The listing builds one solid part. Answer for the finished solid, in the listing's coordinates (mm). A direction names the side the tool comes from. Round coordinates to 2 decimals unless told otherwise and drop trailing zeros. Write each loop counter-clockwise with the first axis right and the second up, starting at its lowest first coordinate (ties: lowest second). Pieces come first, ordered by that corner, then holes.
(1) A cutting plane is placed at A-A, the plane x = 0. Give the vertices of the cut face in (y, z).
(2) Find the intervals of material crossed by probe 1 along X at (y, z) = (0.3, 0); probe 2 along Z at (x, y) = (-4.5, 0.2); probe 3 along Y at (x, z) = (2.5, -3.75), in increasing order.
(3) For faces 1 (the face through (4, 1, -3)), 2 (the face through (-2.583, 0.707, 1.517)), determine the directions among +Z, -Z, +X, -X, +Y, -Y from which every point of the face is accessible in a straight line to the end or side of a thin tool.
(4) A cutting plane is placed at B-B, the plane y = 0.4. Give the vertices of the cut face in (x, z), and give its area (3 significant figures).
(5) A cutting plane is placed at C-C, the plane z = -2.5. Give the number of separate pieces and of enclosed holes in the cut face, and give its area (3 significant figures).
from build123d import *

# Parameters (mm, degrees)
CUT_SLIT_DEPTH         = 9.079913366
PATTERN_CUT_SLIT_COUNT = 6


with BuildPart() as part:
    # Sketch4 → Body-Washer (revolve)
    with BuildSketch(Plane.XY, mode=Mode.PRIVATE) as body_washer_sk:
        with BuildLine():
            Line((1.5, 0.2), (4.45, 1.2))
            Line((4.45, 1.2), (5.45, 1.2))
            ThreePointArc((5.45, 1.2), (5.591421356, 1.141421356), (5.65, 1))
            Line((5.65, 1), (5.65, 0))
            Line((5.65, 0), (5.45, 0))
            Line((5.45, 0), (5.45, 1))
            Line((5.45, 1), (4.482976725, 1))
            Line((4.482976725, 1), (1.564207856, 0.010586824))
            Line((1.564207856, 0.010586824), (1.5, 0.2))
        make_face()
    revolve(body_washer_sk.sketch.rotate(Axis((0, 1.2, 0), (0, -1, 0)), 90), axis=Axis((0, 1.2, 0), (0, -1, 0)))

    # Sketch5 → Cut-Slit (cut, through all)
    with BuildSketch(Plane(origin=(0, 0, 0), x_dir=(1, 0, 0), z_dir=(0, 1, 0))):
        with BuildLine():
            Line((4.091996679, 0.358003321), (1.45665151, 0.358003321))
            ThreePointArc((1.45665151, 0.358003321), (1.5, 0), (1.45665151, -0.358003321))
            Line((1.45665151, -0.358003321), (4.091996679, -0.358003321))
            ThreePointArc((4.091996679, -0.358003321), (4.45, 0), (4.091996679, 0.358003321))
        make_face()
    cut_slit = extrude(amount=CUT_SLIT_DEPTH, mode=Mode.SUBTRACT)

    # Pattern-Cut-Slit: Cut-Slit ×6 about axis
    pattern_cut_slit_axis = Axis((0, 0, 0), (0, 1, 0))
    for i in range(1, PATTERN_CUT_SLIT_COUNT):
        add(cut_slit.rotate(pattern_cut_slit_axis, i * 360 / PATTERN_CUT_SLIT_COUNT), mode=Mode.SUBTRACT)


solid = part.part
Solutions:
1. outline: (0, -5.65) - (1, -5.65) arc R0.2 ccw to (1.2, -5.45) - (1.2, -4.45) - (0.2, -1.5) - (0.01, -1.56) - (1, -4.48) - (1, -5.45) - (0, -5.45) - close; (0, 5.45) - (1, 5.45) - (1, 4.48) - (0.01, 1.56) - (0.2, 1.5) - (1.2, 4.45) - (1.2, 5.45) arc R0.2 ccw to (1, 5.65) - (0, 5.65) - close
2. probe 1: x = -5.65 to -5.45, 5.45 to 5.65
2. probe 2: z = -3.42 to -3.07, 3.07 to 3.42
2. probe 3: y = 1 to 1.2
3. face 1: -Y
3. face 2: +Y
4. outline: circle Ø11.3 at (0, 0); (-2.69, -0.36) arc R2.71 ccw to (-1.65, -2.15) - (-1.34, -1.6) arc R2.09 cw to (-2.06, -0.36) - close; (-2.69, 0.36) - (-2.06, 0.36) arc R2.09 cw to (-1.34, 1.6) - (-1.65, 2.15) arc R2.71 ccw to start; (-1.03, -2.51) arc R2.71 ccw to (1.03, -2.51) - (0.72, -1.96) arc R2.09 cw to (-0.72, -1.96) - close; (-1.03, 2.51) - (-0.72, 1.96) arc R2.09 cw to (0.72, 1.96) - (1.03, 2.51) arc R2.71 ccw to start; (1.34, -1.6) - (1.65, -2.15) arc R2.71 ccw to (2.69, -0.36) - (2.06, -0.36) arc R2.09 cw to start; (1.34, 1.6) arc R2.09 cw to (2.06, 0.36) - (2.69, 0.36) arc R2.71 ccw to (1.65, 2.15) - close; hole circle Ø10.9 at (0, 0)
4. area: 13.7 mm2
5. separate pieces: 3
5. enclosed holes: 0
5. area: 2.19 mm2
